```python
from build123d import *

# Parameters (mm, degrees)
F0_R     = 10
F1_DEPTH = 8
F2_R     = 17.5
F3_DEPTH = 14
F4_R     = 5
F5_DEPTH = 40


with BuildPart() as f1:
    # F0 (on Top) → F1 (new body)
    with BuildSketch(Plane.XY):
        Circle(F0_R)
    extrude(amount=F1_DEPTH)

    # F2 (on face) → F3 (join)
    with BuildSketch(Plane.XY.offset(8)):
        Circle(F2_R)
    extrude(amount=F3_DEPTH)

    # F4 (on face) → F5 (cut)
    with BuildSketch(Plane.XY.offset(22)):
        Circle(F4_R)
    extrude(amount=-F5_DEPTH, mode=Mode.SUBTRACT)


solid = f1.part
```
Read the model definition and answer for the solid it produces. Units are mm, in the model's axes. A direction names the side the tool comes from. Give positions to 0.01 mm unless a question says otherwise; leave off trailing zeros. Order: outer loops, then holes, each group sorted by start corner. A loop starts at its lowest first (then second) coordinate and runs counter-clockwise, first axis right, second up.
(1) Find section D-D (x = -6). Give the vertices of the cut face in (y, z), plus the area to 3 significant figures.
(2) Find section A-A (y = 0). Give the vertices of the cut face in (x, z), plus the area to 3 significant figures.
(3) For a pull along Y with two mould halves and no side action, classify faces 1 (the flat face through (-5, -2, 0)), 2 (the cylindrical face through (-13.887, -10.648, 14.902)), 3 (the cylindrical face through (-1.08, -4.88, 11.15)) as released by +Y, released by -Y, zero draft, split by the parting line, or undercut.
(4) Given pin 1 (3 mm diameter, centred on x = -5.5, z = 15.5, fed in from +Y); pin 2 (2 mm diameter, centred on x = 9.5, z = 4.5, fed in from +Y); pin 3 (1.5 mm diameter, centred on y = -3.5, z = 10.5, fed in from -X), each flat-ended and moving along its own axis, determine where each tip first touches the part or whether it passes through.
(5) For faces 4 (the flat face through (4, -4, 22)), 5 (the flat face through (8, -8, 8)), determine the directions among +Z, -Z, +X, -X, +Y, -Y from which every point of the face is accessible in a straight line to the end or side of a thin tool.
(6) Straight lines are drawn through the part: L1, parallel to Y at x = 0, z = 7.75; L2, parallel to Y at x = 0, z = 10; L3, parallel to X at y = -4, z = 10. For each, find the intervals that lie inside material, in ascending order.
(7) Find section C-C (z = 17). Give the vertices of the cut face in (x, y).
Result sheet:
1. outline: (-16.44, 8) - (-8, 8) - (-8, 0) - (8, 0) - (8, 8) - (16.44, 8) - (16.44, 22) - (-16.44, 22) - close
1. area: 588 mm2
2. outline: (-17.5, 8) - (-10, 8) - (-10, 0) - (-5, 0) - (-5, 22) - (-17.5, 22) - close; (5, 0) - (10, 0) - (10, 8) - (17.5, 8) - (17.5, 22) - (5, 22) - close
2. area: 430 mm2
3. face 1: zero draft
3. face 2: split by the parting line
3. face 3: undercut
4. pin 1: stops at y = 17.04
4. pin 2: stops at y = 5.27
4. pin 3: stops at x = -17.28
5. face 4: +Z, +X, -X, +Y, -Y
5. face 5: -Z
6. L1: y = -10 to -5, 5 to 10
6. L2: y = -17.5 to -5, 5 to 17.5
6. L3: x = -17.04 to -3, 3 to 17.04
7. outline: circle Ø35 at (0, 0); hole circle Ø10 at (0, 0)
